Work out the finished part from the listing and answer in its coordinate system (mm). A direction names the side the tool comes from. Coordinates: 2 decimals unless noted, no trailing zeros. Order: outer loops, then holes, each group sorted by start corner. A loop starts at its lowest first (then second) coordinate and runs counter-clockwise, first axis right, second up. Notation, with made-up numbers: M 33.5,14 L 39.5,14 A25 ccw 39.5,37 Z; hole C 76.5,30.5 d1. An arc over 180 degrees is marked long. Use a Markdown table: item, result.
Autodesk Inventor part; units mm, degrees
ref_plane "YZ Plane" through (0, 0, 0) normal (1, 0, 0) x (0, 1, 0)
ref_plane "XZ Plane" through (0, 0, 0) normal (0, 1, 0) x (-1, 0, 0)
ref_plane "XY Plane" through (0, 0, 0) normal (0, 0, 1) x (1, 0, 0)
sketch "Sketch2" plane through (0, 0, 0) normal (0, 0, 1) x (1, 0, 0)
  line L0 (0, 0) -> (0, 3.175)
  line L1 (0, 3.175) -> (50.8, 3.175)
  line L2 (50.8, 3.175) -> (53.975, 3.175)
  line L3 (53.975, 3.175) -> (53.975, -123.825)
  line L4 (53.975, -123.825) -> (108.712, -123.825)
  line L5 (108.712, -123.825) -> (163.449, -123.825)
  line L6 (163.449, -123.825) -> (166.624, -123.825)
  line L7 (166.624, -123.825) -> (166.624, -127)
  line L8 (166.624, -127) -> (166.624, -165.1)
  line L9 (166.624, -165.1) -> (166.624, -168.275)
  line L10 (166.624, -168.275) -> (163.449, -168.275)
  line L11 (163.449, -168.275) -> (0, -168.275)
  line L12 (0, -168.275) -> (-3.175, -168.275)
  line L13 (-3.175, -168.275) -> (-3.175, 0)
  line L14 (-3.175, 0) -> (-3.175, 3.175)
  line L15 (-3.175, 3.175) -> (0, 3.175)
  dimension "d6" = 3.175
  dimension "d13" = 3.175
  dimension "d16" = 3.175
extrude "Extrusion1" add sketch "Sketch2" along normal blind 55.5625
shell "Shell1" thickness 3.175 removed faces 1 at (15.875, -97.3667, 55.5625)
sketch "Sketch3" plane through (0, -165.1, 3.175) normal (0, 0, 1) x (1, 0, 0)
  line L0 (50.8, 38.1) -> (163.449, 38.1)
  line L1 (163.449, 0) -> (0, 0)
  line L2 (50.8, 38.1) -> (53.975, 38.1)
  line L3 (53.975, 38.1) -> (53.975, 0)
  line L4 (53.975, 0) -> (50.8, 0)
  line L5 (50.8, 0) -> (50.8, 38.1)
  point P0 (0, 165.1)
  dimension "d21" = 3.175
extrude "Extrusion2" add sketch "Sketch3" along normal blind 38.1
sketch "Sketch4" plane through (0, 0, 3.175) normal (0, 0, 1) x (1, 0, 0)
  line L0 (0, 0) -> (50.8, 0)
  line L1 (0, 0) -> (6.8, 0)
  line L2 (6.8, 0) -> (6.8, -6.8)
  line L3 (6.8, -6.8) -> (0, -6.8)
  line L4 (0, -6.8) -> (0, 0)
  line L5 (50.8, 0) -> (44, 0)
  line L6 (44, 0) -> (44, -6.8)
  line L7 (44, -6.8) -> (50.8, -6.8)
  line L8 (50.8, -6.8) -> (50.8, 0)
  line L9 (0, -165.1) -> (0, 0)
  line L10 (0, -165.1) -> (6.8, -165.1)
  line L11 (6.8, -165.1) -> (6.8, -158.3)
  line L12 (6.8, -158.3) -> (0, -158.3)
  line L13 (0, -158.3) -> (0, -165.1)
  line L14 (50.8, -127) -> (163.449, -127)
  line L15 (53.9685, -127) -> (62.7685, -127)
  line L16 (62.7685, -127) -> (62.7685, -133.8)
  line L17 (62.7685, -133.8) -> (53.9685, -133.8)
  line L18 (53.9685, -133.8) -> (53.9685, -127)
  line L19 (163.449, -127) -> (163.449, -165.1)
  line L20 (163.449, -127) -> (156.649, -127)
  line L21 (156.649, -127) -> (156.649, -133.8)
  line L22 (156.649, -133.8) -> (163.449, -133.8)
  line L23 (163.449, -133.8) -> (163.449, -127)
  line L24 (163.449, -165.1) -> (156.649, -165.1)
  line L25 (156.649, -165.1) -> (156.649, -158.3)
  line L26 (156.649, -158.3) -> (163.449, -158.3)
  line L27 (163.449, -158.3) -> (163.449, -165.1)
extrude "Extrusion3" add sketch "Sketch4" along normal blind 50.8
sketch "Sketch5" plane through (0, 0, 53.975) normal (0, 0, 1) x (1, 0, 0)
  line L0 (0, -165.1) -> (0, 0)
  line L1 (0, 0) -> (2.15, 0)
  line L2 (2.15, 0) -> (2.15, -2.15)
  line L3 (2.15, -2.15) -> (0, -2.15)
  line L4 (0, -2.15) -> (0, 0)
  line L5 (50.8, 0) -> (50.8, -127)
  line L6 (50.8, 0) -> (48.65, 0)
  line L7 (48.65, 0) -> (48.65, -2.15)
  line L8 (48.65, -2.15) -> (50.8, -2.15)
  line L9 (50.8, -2.15) -> (50.8, 0)
  line L10 (163.449, -165.1) -> (0, -165.1)
  line L11 (0, -165.1) -> (2.15, -165.1)
  line L12 (2.15, -165.1) -> (2.15, -162.95)
  line L13 (2.15, -162.95) -> (0, -162.95)
  line L14 (0, -162.95) -> (0, -165.1)
  line L15 (53.9685, -127) -> (53.9685, -133.8)
  line L16 (53.9685, -127) -> (58.3685, -127)
  line L17 (62.7685, -133.8) -> (62.7685, -127)
  line L18 (58.3685, -127) -> (58.3685, -129.15)
  line L19 (50.8, -127) -> (163.449, -127)
  line L20 (163.449, -127) -> (161.299, -127)
  line L21 (161.299, -127) -> (161.299, -129.15)
  line L22 (161.299, -129.15) -> (163.449, -129.15)
  line L23 (163.449, -129.15) -> (163.449, -127)
  line L24 (163.449, -127) -> (163.449, -165.1)
  line L25 (163.449, -165.1) -> (161.299, -165.1)
  line L26 (161.299, -165.1) -> (161.299, -162.95)
  line L27 (161.299, -162.95) -> (163.449, -162.95)
  line L28 (163.449, -162.95) -> (163.449, -165.1)
hole "Hole1" at (2.15, -2.15, 53.975) at (48.65, -2.15, 53.975) at (2.15, -162.95, 53.975) at (58.3685, -129.15, 53.975) at (161.299, -129.15, 53.975) at (161.299, -162.95, 53.975) direction (0, 0, -1) diameter 3.5 depth 3.5
fillet "Fillet1" radius 2 5 edges at (53.975, 3.175, 27.7812) (166.624, -123.825, 27.7812) (166.624, -168.275, 27.7812) (-3.175, -168.275, 27.7812) (-3.175, 3.175, 27.7812)
fillet "Fillet2" radius 2 7 edges at (6.8, -158.3, 28.575) (6.8, -6.8, 28.575) (44, -6.8, 28.575) (62.7685, -133.8, 28.575) (53.9685, -133.8, 47.625) (156.649, -158.3, 28.575) (156.649, -133.8, 28.575)
sketch "Sketch6" plane through (53.975, -123.825, 55.5625) normal (1, 0, 0) x (0, 0, -1)
  line L0 (52.3875, 123.825) -> (1.5875, 123.825)
  line L1 (52.3875, 123.825) -> (52.3875, 88.825)
  line L2 (52.3875, -34.475) -> (52.3875, 117.025)
  line L3 (52.3875, 88.825) -> (26.9875, 88.825)
  line L4 (0, 123.825) -> (0, -3.175)
  point P0 (55.5625, 123.825)
  dimension "d58" = 35
  dimension "d59" = 25.4
hole "Hole2" at (53.975, -35, 28.575) direction (-1, 0, 0) diameter 22 depth 3.175
sketch "Sketch7" plane through (53.975, -123.825, 55.5625) normal (0, 1, 0) x (1, 0, 0)
  line L0 (0, 52.3875) -> (0, 14.2875)
  line L1 (0, 52.3875) -> (54.737, 52.3875)
  line L2 (102.674, 52.3875) -> (0, 52.3875)
  line L3 (54.737, 52.3875) -> (54.737, 26.9875)
  point P0 (-53.975, 55.5625)
  dimension "d67" = 54.737
  dimension "d68" = 25.4
hole "Hole3" at (108.712, -123.825, 28.575) direction (0, -1, 0) diameter 15.5 end through all
sketch "Sketch8" plane through (53.975, -123.825, 55.5625) normal (1, 0, 0) x (0, 0, -1)
  circle A0 centre (26.9875, 88.825) radius 11
  line L0 (26.9875, 88.825) -> (26.9875, 106.275)
  line L1 (26.9875, 88.825) -> (42.0996, 80.1)
  line L2 (26.9875, 88.825) -> (44.4375, 88.825) construction
  line L3 (26.9875, 88.825) -> (11.8754, 80.1)
  line L4 (26.9875, 88.825) -> (44.4375, 88.825) construction
  point P0 (55.5625, 123.825)
  dimension "d76" = 17.45
  dimension "d77" = 17.45
  dimension "d78" = 30
  dimension "d79" = 17.45
  dimension "d80" = 150
hole "Hole4" at (53.975, -17.55, 28.575) at (53.975, -43.725, 13.4629) at (53.975, -43.725, 43.6871) direction (-1, 0, 0) diameter 3.5 depth 3.175
sketch "Sketch9" plane through (-3.175, -166.275, 0) normal (-1, 0, 0) x (0, 0, 1)
  circle A0 centre (28.575, 131.275) radius 11
  line L0 (28.575, 146.775) -> (13.075, 146.775)
  line L1 (13.075, 146.775) -> (44.075, 146.775)
  line L2 (44.075, 146.775) -> (44.075, 115.775)
  line L3 (44.075, 115.775) -> (13.075, 115.775)
  line L4 (13.075, 115.775) -> (13.075, 146.775)
  point P0 (0, 166.275)
  dimension "d90" = 31
  dimension "d91" = 31
hole "Hole5" at (-3.175, -50.5, 13.075) at (-3.175, -19.5, 13.075) at (-3.175, -19.5, 44.075) at (-3.175, -50.5, 44.075) direction (1, 0, 0) diameter 3 depth 3.175
sketch "Sketch10" plane through (50.8, -127, 55.5625) normal (-1, 0, 0) x (0, 0, 1)
  line L0 (-14.2875, -38.1) -> (-52.3875, -38.1)
  line L1 (-52.3875, -38.1) -> (-38.2875, -38.1)
  line L2 (-38.2875, -38.1) -> (-38.2875, -24)
  line L3 (-38.2875, -24) -> (-38.2875, -12.5)
  line L4 (-38.2875, -12.5) -> (-49.7875, -12.5)
  line L5 (-49.7875, -12.5) -> (-26.7875, -12.5)
  line L6 (-26.7875, -12.5) -> (-26.7875, -35.5)
  line L7 (-26.7875, -35.5) -> (-49.7875, -35.5)
  line L8 (-49.7875, -35.5) -> (-49.7875, -12.5)
  point P0 (-55.5625, 127)
  dimension "d99" = 14.1
  dimension "d100" = 14.1
  dimension "d101" = 11.5
  dimension "d102" = 11.5
  dimension "d103" = 23
  dimension "d104" = 23
hole "Hole6" at (50.8, -139.5, 5.775) at (50.8, -139.5, 28.775) at (50.8, -162.5, 28.775) at (50.8, -162.5, 5.775) direction (1, 0, 0) diameter 2.5 depth 3.175
sketch "Sketch11" plane through (166.624, -166.275, 0) normal (1, 0, 0) x (0, 0, -1)
  line L0 (-53.975, 39.275) -> (-53.975, 34.475)
  line L1 (-53.975, 39.275) -> (-49.575, 39.275)
  line L2 (-3.175, 39.275) -> (-53.975, 39.275)
  line L3 (-49.575, 39.275) -> (-49.575, 37.125)
  line L4 (-50.475, 38.875) -> (-50.475, 35.375)
  line L5 (-3.175, 34.475) -> (-3.175, 39.275)
  line L6 (-3.175, 39.275) -> (-7.575, 39.275)
  line L7 (-7.575, 39.275) -> (-7.575, 37.125)
  line L8 (-53.975, 1.175) -> (-3.175, 1.175)
  line L9 (-53.975, 1.175) -> (-49.575, 1.175)
  line L10 (-49.575, 1.175) -> (-49.575, 3.325)
  line L11 (-3.175, 1.175) -> (-3.175, 5.975)
  line L12 (-3.175, 1.175) -> (-7.575, 1.175)
  line L13 (-7.575, 1.175) -> (-7.575, 3.325)
  point P0 (0, 166.275)
  dimension "d112" = 4.4
  dimension "d113" = 2.15
  dimension "d114" = 90
  dimension "d115" = 4.4
  dimension "d116" = 2.15
  dimension "d117" = 4.4
  dimension "d118" = 2.15
  dimension "d119" = 4.4
  dimension "d120" = 2.15
hole "Hole7" at (166.624, -129.15, 49.575) at (166.624, -129.15, 7.575) at (166.624, -162.95, 49.575) at (166.624, -162.95, 7.575) direction (-1, 0, 0) diameter 3.5 depth 3.175
fillet "Fillet3" radius 2 2 edges at (50.8, -127, 48.4188) (53.975, -123.825, 27.7812)
properties part number "Main Lidar Body-01"
(1) A cutting plane is placed at B-B (y = -11). Determine the outline of the cut face in (x, z) (1 decimal).
Conclusion:
| item | result |
|---|---|
| outline | M -3.2,0 L 54,0 L 54,55.6 L 50.8,55.6 L 50.8,3.2 L 0,3.2 L 0,55.6 L -3.2,55.6 Z |
(2) Given P1, Ø2, axis at x = 132.5, z = 25, coming from the +Y side (3 decimals); P2, Ø1.7, axis at y = -128.5, z = 7, coming from the +X side; P3, Ø1.5, axis at x = 19.5, y = -141.5, coming from the +Z side (3 decimals), each flat-ended and moving along its own axis, determine where each tip first touches the part or whether it passes through.
Conclusion:
| item | result |
|---|---|
| P1 | y = -123.825 |
| P2 | x = 163.45 |
| P3 | z = 3.175 |
(3) Straight lines are drawn through the part: L1, parallel to X at y = -131, z = 9.5 (1 decimal); L2, parallel to Y at x = 144.5, z = 40.5 (3 decimals); L3, parallel to Y at x = 23, z = 30 (3 decimals). For each, find the intervals that lie inside material, in ascending order.
Conclusion:
| item | result |
|---|---|
| L1 | -3.2 to 0, 50.8 to 62.8, 156.6 to 166.6 |
| L2 | -168.275 to -165.1, -127 to -123.825 |
| L3 | -168.275 to -165.1, 0 to 3.175 |
(4) Which of the six approach directions +Z, -Z, +X, -X, +Y, -Y give full straight-line access (tool end or side, diameter ignored) to faces 1 (the flat face through (-3.175, -84, 27)), 2 (the flat face through (58.3, -131.1, 53.975)), 3 (the flat face through (53.975, -59, 27))?
Conclusion:
| item | result |
|---|---|
| face 1 | +Z, -Z, -X, +Y, -Y |
| face 2 | +Z |
| face 3 | +Z, -Z, +X, +Y |
(5) A cutting plane is placed at A-A (x = 70). Determine the outline of the cut face in (y, z) (1 decimal), then the cut area to 3 significant figures.
Conclusion:
| item | result |
|---|---|
| outline | M -168.3,0 L -123.8,0 L -123.8,55.6 L -127,55.6 L -127,3.2 L -165.1,3.2 L -165.1,55.6 L -168.3,55.6 Z |
| area | 474 mm2 |
(6) A cutting plane is placed at C-C (y = -143.5). Determine the outline of the cut face in (x, z) (1 decimal).
Conclusion:
| item | result |
|---|---|
| outline | M -3.2,0 L 166.6,0 L 166.6,55.6 L 163.4,55.6 L 163.4,3.2 L 54,3.2 L 54,41.3 L 50.8,41.3 L 50.8,3.2 L 0,3.2 L 0,55.6 L -3.2,55.6 Z |
(7) Determine the mould class of faces 4 (the flat face through (83, -168.275, 27)), 5 (the cylindrical face through (116.278, -125.435, 26.895)), 6 (the flat face through (108, -146, 3.175)) for opening direction Y: pulls with the +Y half, pulls with the -Y half, needs draft (parallel to the pull), parting line crosses it, or undercut.
Conclusion:
| item | result |
|---|---|
| face 4 | pulls with the -Y half |
| face 5 | needs draft |
| face 6 | undercut |
